Autodesk Inventor part; units mm, degrees
ref_plane "YZ Plane" through (0, 0, 0) normal (1, 0, 0) x (0, 1, 0)
ref_plane "XZ Plane" through (0, 0, 0) normal (0, 1, 0) x (-1, 0, 0)
ref_plane "XY Plane" through (0, 0, 0) normal (0, 0, 1) x (1, 0, 0)
sketch "Sketch1" plane through (0, 0, 0) normal (0, 0, 1) x (1, 0, 0)
  circle A0 centre (0, 0) radius 15
  arc A1 (-2.6749, 24.8565) -> (-12.4462, 21.6816) centre (0, 0) ccw
  arc A2 (-16.7743, 18.5371) -> (-22.8133, 10.2251) centre (0, 0) ccw
  arc A3 (12.4462, 21.6816) -> (2.6749, 24.8565) centre (0, 0) ccw
  arc A4 (22.8133, 10.2251) -> (16.7743, 18.5371) centre (0, 0) ccw
  arc A5 (24.4665, -5.1371) -> (24.4665, 5.1371) centre (0, 0) ccw
  arc A6 (16.7743, -18.5371) -> (22.8133, -10.2251) centre (0, 0) ccw
  arc A7 (2.6749, -24.8565) -> (12.4462, -21.6816) centre (0, 0) ccw
  arc A8 (-12.4462, -21.6816) -> (-2.6749, -24.8565) centre (0, 0) ccw
  arc A9 (-22.8133, -10.2251) -> (-16.7743, -18.5371) centre (0, 0) ccw
  arc A10 (-24.4665, 5.1371) -> (-24.4665, -5.1371) centre (0, 0) ccw
  line L0 (-16.7743, 18.5371) -> (-20.306, 24.7319)
  line L1 (-20.306, 24.7319) -> (-18.8091, 25.8885)
  line L2 (-18.8091, 25.8885) -> (-17.2465, 26.9547)
  line L3 (-17.2465, 26.9547) -> (-12.4462, 21.6816)
  line L4 (-24.4665, 5.1371) -> (-30.9649, 8.0729)
  line L5 (-30.9649, 8.0729) -> (-30.4338, 9.8885)
  line L6 (-30.4338, 9.8885) -> (-29.7963, 11.6696)
  line L7 (-29.7963, 11.6696) -> (-22.8133, 10.2251)
  line L8 (-22.8133, -10.2251) -> (-29.7963, -11.6696)
  line L9 (-29.7963, -11.6696) -> (-30.4338, -9.8885)
  line L10 (-30.4338, -9.8885) -> (-30.9649, -8.0729)
  line L11 (-30.9649, -8.0729) -> (-24.4665, -5.1371)
  line L12 (-12.4462, -21.6816) -> (-17.2465, -26.9547)
  line L13 (-17.2465, -26.9547) -> (-18.8091, -25.8885)
  line L14 (-18.8091, -25.8885) -> (-20.306, -24.7319)
  line L15 (-20.306, -24.7319) -> (-16.7743, -18.5371)
  line L16 (2.6749, -24.8565) -> (1.8909, -31.9441)
  line L17 (1.8909, -31.9441) -> (0, -32)
  line L18 (0, -32) -> (-1.8909, -31.9441)
  line L19 (-1.8909, -31.9441) -> (-2.6749, -24.8565)
  line L20 (16.7743, -18.5371) -> (20.306, -24.7319)
  line L21 (20.306, -24.7319) -> (18.8091, -25.8885)
  line L22 (18.8091, -25.8885) -> (17.2465, -26.9547)
  line L23 (17.2465, -26.9547) -> (12.4462, -21.6816)
  line L24 (24.4665, -5.1371) -> (30.9649, -8.0729)
  line L25 (30.9649, -8.0729) -> (30.4338, -9.8885)
  line L26 (30.4338, -9.8885) -> (29.7963, -11.6696)
  line L27 (29.7963, -11.6696) -> (22.8133, -10.2251)
  line L28 (22.8133, 10.2251) -> (29.7963, 11.6696)
  line L29 (29.7963, 11.6696) -> (30.4338, 9.8885)
  line L30 (30.4338, 9.8885) -> (30.9649, 8.0729)
  line L31 (30.9649, 8.0729) -> (24.4665, 5.1371)
  line L32 (12.4462, 21.6816) -> (17.2465, 26.9547)
  line L33 (17.2465, 26.9547) -> (18.8091, 25.8885)
  line L34 (18.8091, 25.8885) -> (20.306, 24.7319)
  line L35 (20.306, 24.7319) -> (16.7743, 18.5371)
  line L36 (-2.6749, 24.8565) -> (-1.8909, 31.9441)
  line L37 (-1.8909, 31.9441) -> (0, 32)
  line L38 (0, 32) -> (1.8909, 31.9441)
  line L39 (1.8909, 31.9441) -> (2.6749, 24.8565)
  point P0 (-2.6749, 24.8565)
  point P1 (-12.4462, 21.6816)
  point P2 (-16.7743, 18.5371)
  point P3 (-22.8133, 10.2251)
  point P4 (-24.4665, -5.1371)
  point P5 (-22.8133, -10.2251)
  point P6 (-16.7743, -18.5371)
  point P7 (-12.4462, -21.6816)
  point P8 (-2.6749, -24.8565)
  point P9 (12.4462, -21.6816)
  point P10 (16.7743, -18.5371)
  point P11 (22.8133, -10.2251)
  point P12 (24.4665, 5.1371)
  point P13 (22.8133, 10.2251)
  point P14 (16.7743, 18.5371)
  point P15 (12.4462, 21.6816)
  point P16 (2.6749, 24.8565)
extrude "Extrusion1" add sketch "Sketch1" along normal blind 20
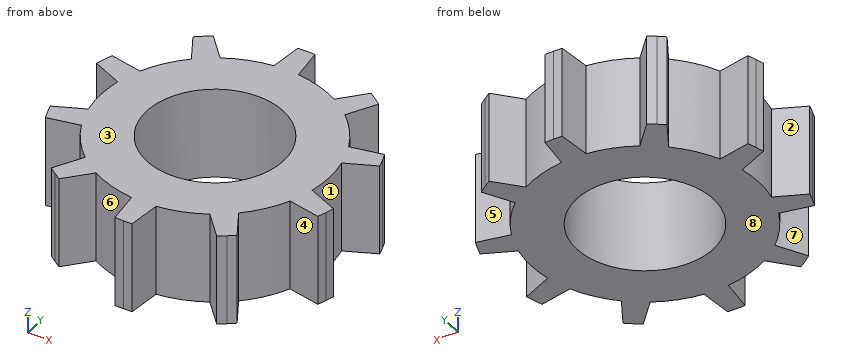
Model file for the job. Use its own axes, mm. Face numbers are marked on the shaded views. A direction names the side the tool comes from. Give positions to 0.01 mm unless a question says otherwise; leave off trailing zeros. Loops run counter-clockwise (first coordinate to the right, second up) from the corner with the lowest first, then second, coordinate; pieces in that order, holes last. Notation, with made-up numbers: (-33, 26.25) -> (-19, 26.25) arc R21 cw to (-19, 59.25) -> close; hole circle Ø7 at (25, 54.25). An arc over 180 degrees is marked (long way). Write each question's results on one line, items separated by ' | '.
(1) Probe line 1 along Y through (x, z) = (0, 10.5); line 2 along Y through (x, z) = (19, 15); line 3 along Y through (x, z) = (-18, 7.75). List the from-to ranges inside material, lowest first.
Geometry results:
line 1: y = -32 to -15, 15 to 32 | line 2: y = -25.74 to -22.44, -16.25 to 16.25, 22.44 to 25.74 | line 3: y = -26.44 to -20.69, -17.35 to 17.35, 20.69 to 26.44
(2) Pull direction X, two halves, no side cores. Call the marked faces 1, 2, 3 and 4: released by +X, released by -X, zero draft, split by the parting line, or undercut.
Geometry results:
face 1: released by +X | face 2: released by -X | face 3: zero draft | face 4: undercut
(3) Cut at B-B on x = -9.5. List the corners of the cut face in (y, z), and give its area (3 significant figures).
Geometry results:
outline: (-23.12, 0) -> (-11.61, 0) -> (-11.61, 20) -> (-23.12, 20) -> close; (11.61, 0) -> (23.12, 0) -> (23.12, 20) -> (11.61, 20) -> close | area: 461 mm²
(4) Tool access for the marked faces 5, 6, 7 and 8: list every direction of +Z, -Z, +X, -X, +Y, -Y with a clear straight run to the whole face (end or side of a thin tool).
Geometry results:
face 5: +Z, -Z, +Y | face 6: +Z, -Z, -Y | face 7: +Z, -Z, -X | face 8: -Z, +X, -X, +Y, -Y
(5) Cut at C-C on y = 23. List the corners of the cut face in (x, z).
Geometry results:
outline: (-19.32, 0) -> (-13.65, 0) -> (-13.65, 20) -> (-19.32, 20) -> close; (-9.8, 0) -> (9.8, 0) -> (9.8, 20) -> (-9.8, 20) -> close; (13.65, 0) -> (19.32, 0) -> (19.32, 20) -> (13.65, 20) -> close
(6) Cut at A-A on y = 0. List the corners of the cut face in (x, z).
Geometry results:
outline: (-25, 0) -> (-15, 0) -> (-15, 20) -> (-25, 20) -> close; (15, 0) -> (25, 0) -> (25, 20) -> (15, 20) -> close
(7) Flat gauge pins, fed straight in: pin 1 Ø3 at (y, z) = (-22, 7.5) entering from -X; pin 2 Ø10 at (x, z) = (-21.5, 7) entering from +Y; pin 3 Ø5 at (y, z) = (-2.5, 15) entering from +X. Where does each tip first touch, or does it go through?
Geometry results:
pin 1: stops at x = -19.6 | pin 2: stops at y = 26.95 | pin 3: stops at x = 25
